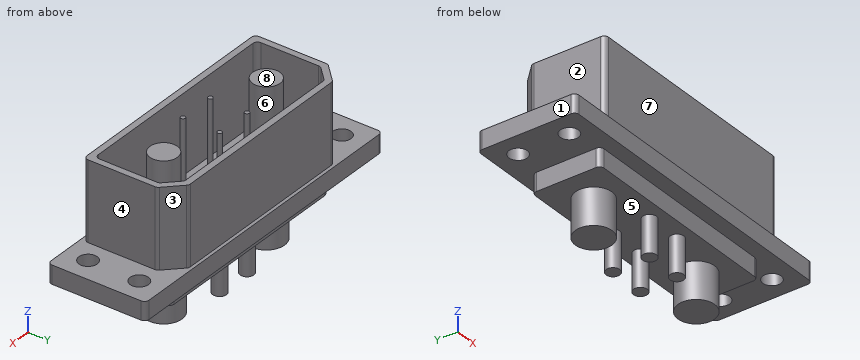
```python
from build123d import *

# Parameters (mm, degrees)
SKETCH_1_W          = 34.6
SKETCH_1_H          = 10.7
EXTRUDE_1_DEPTH     = 2
SKETCH_2_R          = 1
CUT_EXTRUDE_1_DEPTH = 2
EXTRUDE_2_DEPTH     = 8.6
CUT_EXTRUDE_2_DEPTH = 8.5
SKETCH_5_R          = 1.5
SKETCH_5_R_2        = 0.25
EXTRUDE_3_DEPTH     = 8.5
SKETCH_6_W          = 23
SKETCH_6_H          = 7.5
EXTRUDE_4_DEPTH     = 2
SKETCH_7_R          = 2
SKETCH_7_R_2        = 0.75
EXTRUDE_5_DEPTH     = 4
FILLET_2_R          = 0.5


with BuildPart() as part:
    # 草图1 → 凸台-拉伸1 (new body)
    with BuildSketch(Plane.XY):
        Rectangle(SKETCH_1_W, SKETCH_1_H)
    extrude(amount=EXTRUDE_1_DEPTH)

    # 草图2 → 切除-拉伸1 (cut)
    with BuildSketch(Plane.XY.offset(2)):
        with Locations((-14.8, 2.8)):
            Circle(SKETCH_2_R)
        with Locations(Location((14.8, 2.8, 0), (0, 0, 180))):
            Circle(SKETCH_2_R)
        with Locations((14.8, -2.8)):
            Circle(SKETCH_2_R)
        with Locations(Location((-14.8, -2.8, 0), (0, 0, 180))):
            Circle(SKETCH_2_R)
    extrude(amount=-CUT_EXTRUDE_1_DEPTH, mode=Mode.SUBTRACT)

    # 草图3 → 凸台-拉伸2 (add)
    with BuildSketch(Plane.XY.offset(2)):
        Polygon((10.5, 5), (-10.5, 5), (-12.5, 3), (-12.5, -5), (12.5, -5), (12.5, 3), align=None)
    extrude(amount=EXTRUDE_2_DEPTH)

    # 草图4 → 切除-拉伸2 (cut)
    with BuildSketch(Plane.XY.offset(10.6)):
        Polygon((-10.210050506, 4.3), (-11.8, 2.710050506), (-11.8, -4.3), (11.8, -4.3), (11.8, 2.710050506), (10.210050506, 4.3), align=None)
    extrude(amount=-CUT_EXTRUDE_2_DEPTH, mode=Mode.SUBTRACT)

    # 草图5 → 凸台-拉伸3 (add)
    with BuildSketch(Plane.XY.offset(2.1)):
        with Locations((-7.5, 0)):
            Circle(SKETCH_5_R)
        with Locations((-2, 2)):
            Circle(SKETCH_5_R_2)
        with Locations(Location((2, 2, 0), (0, 0, 180))):
            Circle(SKETCH_5_R_2)
        with Locations(Location((7.5, 0, 0), (0, 0, 180))):
            Circle(SKETCH_5_R)
        with Locations((2, -2)):
            Circle(SKETCH_5_R_2)
        with Locations(Location((-2, -2, 0), (0, 0, 180))):
            Circle(SKETCH_5_R_2)
    extrude(amount=EXTRUDE_3_DEPTH)

    # 草图6 → 凸台-拉伸4 (add)
    with BuildSketch(Plane(origin=(0, 0, 0), x_dir=(-1, 0, 0), z_dir=(0, 0, -1))):
        Rectangle(SKETCH_6_W, SKETCH_6_H)
    extrude(amount=EXTRUDE_4_DEPTH)

    # 草图7 → 凸台-拉伸5 (add)
    with BuildSketch(Plane(origin=(0, 0, -2), x_dir=(-1, 0, 0), z_dir=(0, 0, -1))):
        with Locations(Location((-7.5, 0, 0), (0, 0, 180))):
            Circle(SKETCH_7_R)
        with Locations(Location((-2, 2, 0), (0, 0, 180))):
            Circle(SKETCH_7_R_2)
        with Locations(Location((2, 2, 0), (0, 0, 180))):
            Circle(SKETCH_7_R_2)
        with Locations(Location((7.5, 0, 0), (0, 0, 180))):
            Circle(SKETCH_7_R)
        with Locations(Location((2, -2, 0), (0, 0, 180))):
            Circle(SKETCH_7_R_2)
        with Locations(Location((-2, -2, 0), (0, 0, 180))):
            Circle(SKETCH_7_R_2)
    extrude(amount=EXTRUDE_5_DEPTH)

    # 圆角2
    fillet_2_edges = [part.edges().sort_by_distance(p)[0] for p in [
        (-10.5, 5, 6.3),
        (-12.5, 3, 6.3),
        (-12.5, -5, 6.3),
        (12.5, -5, 6.3),
        (12.5, 3, 6.3),
        (10.5, 5, 6.3),
        (-10.210050506, 4.3, 6.35),
        (10.210050506, 4.3, 6.35),
        (11.8, 2.710050506, 6.35),
        (11.8, -4.3, 6.35),
        (-11.8, -4.3, 6.35),
        (-11.8, 2.710050506, 6.35),
        (17.3, -5.35, 1),
        (-17.3, -5.35, 1),
        (-17.3, 5.35, 1),
        (17.3, 5.35, 1),
        (-11.5, -3.75, -1),
        (-11.5, 3.75, -1),
        (11.5, 3.75, -1),
        (11.5, -3.75, -1),
    ]]
    fillet(fillet_2_edges, radius=FILLET_2_R)


solid = part.part
```
The listing builds one solid part. Answer for the finished solid, in the listing's coordinates (mm). Face numbers are marked on the shaded views. A direction names the side the tool comes from. Round coordinates to 2 decimals unless told otherwise and drop trailing zeros. Order: outer loops, then holes, each group sorted by start corner. A loop starts at its lowest first (then second) coordinate and runs counter-clockwise, first axis right, second up. Notation, with made-up numbers: (-39.75, -3) - (0.25, -3) arc R16 ccw to (0.25, 9) - close; hole circle Ø7 at (4, 15.25). An arc over 180 degrees is marked (long way). Put each result on its own line as item: value. Start each with the question number.
(1) Given P1, Ø1, axis at y = -0.5, z = -1, coming from the -X side; P2, Ø3, axis at x = -0.5, y = -1, coming from the +Z side; P3, Ø9.5, axis at x = 3.5, z = 7, coming from the +Y side, each flat-ended and moving along its own axis, determine where each tip first touches the part or whether it passes through.
(2) Find section B-B (z = -3). Give the vertices of the cut face in (x, y), plus the area to 3 significant figures.
(3) Find section A-A (z = 2.5). State how many separate pieces and enclosed holes the cut face has, plus the area to 3 significant figures.
(4) Determine the mould class of the marked faces 6, 7 and 8 for opening direction Y: released by +Y, released by -Y, zero draft, split by the parting line, or undercut.
(5) For the marked faces 1, 2, 3, 4 and 5, determine the directions among +Z, -Z, +X, -X, +Y, -Y from which every point of the face is accessible in a straight line to the end or side of a thin tool.
(6) Find section C-C (x = 7.5). Give the vertices of the cut face in (y, z), plus the area to 3 significant figures.
(7) Straight lines are drawn through the part: probe 1 along Y at (x, z) = (-14.8, 0.45); probe 2 along X at (y, z) = (-2.5, 7.75); probe 3 along Y at (x, z) = (10, 7.5). For each, find the intervals that lie inside material, in ascending order. Write a range as from..to.
Reply:
1. P1: x = -11.5
1. P2: z = 2.1
1. P3: y = 5
2. outline: circle Ø4 at (-7.5, 0); circle Ø1.5 at (-2, -2); circle Ø1.5 at (-2, 2); circle Ø1.5 at (2, -2); circle Ø1.5 at (2, 2); circle Ø4 at (7.5, 0)
2. area: 32.2 mm^2
3. separate pieces: 7
3. enclosed holes: 1
3. area: 60.5 mm^2
4. face 6: undercut
4. face 7: released by -Y
4. face 8: zero draft
5. face 1: +Z, -Z, -X, +Y, -Y
5. face 2: +Z, -X, +Y, -Y
5. face 3: +Z, +X, +Y
5. face 4: +Z, +X, +Y, -Y
5. face 5: -Z
6. outline: (-5.35, 0) - (-3.75, 0) - (-3.75, -2) - (-2, -2) - (-2, -6) - (2, -6) - (2, -2) - (3.75, -2) - (3.75, 0) - (5.35, 0) - (5.35, 2) - (5, 2) - (5, 10.6) - (4.3, 10.6) - (4.3, 2.1) - (1.5, 2.1) - (1.5, 10.6) - (-1.5, 10.6) - (-1.5, 2.1) - (-4.3, 2.1) - (-4.3, 10.6) - (-5, 10.6) - (-5, 2) - (-5.35, 2) - close
6. area: 90.8 mm^2
7. probe 1: -5.35..-3.8, -1.8..1.8, 3.8..5.35
7. probe 2: -12.5..-11.8, 11.8..12.5
7. probe 3: -5..-4.3, 4.3..5
